from build123d import *

# Parameters (mm, degrees)
F1_DEPTH = 25.908
F2_W     = 84.75497365
F2_H     = 46.1407359689
F3_DEPTH = 35.306
F4_W     = 85.4094512761
F4_H     = 12.4350916594
F4_H_2   = 13.7440478429
F5_DEPTH = 44.45
F6_W     = 18.3254014701
F6_H     = 12.4350916594
F6_W_2   = 17.998162657
F6_H_2   = 12.1078519151
F6_W_3   = 19.3071179092
F6_H_3   = 13.7440478429
F7_DEPTH = 58.674
F8_R     = 6.9031193851
F9_DEPTH = 43.942


with BuildPart() as f1:
    # F0 (on Top) → F1 (new body)
    with BuildSketch(Plane.XY):
        Polygon((-13.4168099612, 56.1196766794), (-42.8683459759, 56.1196766794), (-42.8683459759, -55.7961538434), (-13.4168099612, -55.7961538434), (-13.4168099612, -41.0703867674), (12.7623323351, -41.0703867674), (12.7623323351, -55.7961538434), (42.2138683498, -55.7961538434), (42.2138683498, 56.1196766794), (12.7623323351, 56.1196766794), (12.7623323351, 41.0666689277), (-13.4168099612, 41.0666689277), align=None)
    extrude(amount=F1_DEPTH)

    # F2 (on Top) → F3 (join)
    with BuildSketch(Plane.XY):
        with Locations((-0.4908591509, 0.3253789619)):
            Rectangle(F2_W, F2_H)
    extrude(amount=F3_DEPTH)

    # F4 (on Top) → F5 (join)
    with BuildSketch(Plane.XY):
        with Locations((-0.4908572882, 17.1782011166)):
            Rectangle(F4_W, F4_H)
        with Locations((-0.4908572882, -15.5457244255)):
            Rectangle(F4_W, F4_H_2)
    extrude(amount=F5_DEPTH)

    # F6 (on Top) → F7 (join)
    with BuildSketch(Plane.XY):
        with Locations((-33.7056452408, 17.1782011166)):
            Rectangle(F6_W, F6_H)
        with Locations((33.2147870213, 17.3418209888)):
            Rectangle(F6_W_2, F6_H_2)
        with Locations((-33.8692646474, -15.5457244255)):
            Rectangle(F6_W_3, F6_H_3)
        with Locations((33.2147870213, -15.5457244255)):
            Rectangle(F6_W_2, F6_H_3)
    extrude(amount=F7_DEPTH)

    # F8 (on Top) → F9 (cut)
    with BuildSketch(Plane.XY):
        with Locations((6.05578674, 0)):
            Circle(F8_R)
    extrude(amount=F9_DEPTH, mode=Mode.SUBTRACT)


solid = f1.part
Check sheet for the modelled part. Datum: model origin and axes. Units: mm. A direction names the side the tool comes from. Round coordinates to 2 decimals unless told otherwise and drop trailing zeros. Order: outer loops, then holes, each group sorted by start corner. A loop starts at its lowest first (then second) coordinate and runs counter-clockwise, first axis right, second up.
(1) Go/stop test with flat-tipped pins: P1, Ø10, axis at x = 11, z = 14, coming from the +Y side; P2, Ø21.5, axis at x = 12.5, y = 2, coming from the +Z side; P3, Ø6, axis at y = 19.5, z = 33, coming from the -X side; P4, Ø16.5, axis at y = 48, z = 13.5, coming from the -X side. Record where each tip stops, or that it passes through.
(2) Cross-section at C-C, the plane x = 34. Enter the section's corners in (y, z), and give its area (3 significant figures).
(3) Cross-section at A-A, the plane y = 0. Enter the section's corners in (x, z), and give its area (3 significant figures).
(4) Cross-section at D-D, the plane z = 11.5. Enter the section's corners in (x, y), and give its area (3 significant figures).
(5) Scan lines: probe 1 along Y at (x, z) = (32, 38); probe 2 along X at (y, z) = (0, 17); probe 3 along Z at (x, y) = (21.5, 40.5). Record each from-to range of solid material in increasing order.
(6) Access from +Z, -Z, +X, -X, +Y, -Y to the whole of each face (thin tool, end or side, straight path). Record for faces 1 (the flat face through (-42.868, 1, 17)), 2 (the flat face through (12.762, -48, 13)), 3 (the flat face through (-42.868, 17, 51)), 4 (the flat face through (33, 11.288, 51)).
(7) Cross-section at B-B, the plane z = 47.5. Enter the section's corners in (x, y), and give its area (3 significant figures).
(8) Draft check along X on faces 5 (the flat face through (24.216, 17, 51)), 6 (the flat face through (-42.868, -39, 13)), 7 (the flat face through (-1, 1, 0)). Enter one of: pulls with the +X half, pulls with the -X half, needs draft (parallel to the pull), parting line crosses it, or undercut.
Check sheet entries:
1. P1: stops at y = 56.12
1. P2: stops at z = 44.45
1. P3: stops at x = -43.2
1. P4: stops at x = -42.87
2. outline: (-55.8, 0) - (56.12, 0) - (56.12, 25.91) - (23.4, 25.91) - (23.4, 58.67) - (11.29, 58.67) - (11.29, 44.45) - (10.96, 44.45) - (10.96, 35.31) - (-8.67, 35.31) - (-8.67, 58.67) - (-22.42, 58.67) - (-22.42, 35.31) - (-22.74, 35.31) - (-22.74, 25.91) - (-55.8, 25.91) - close
2. area: 3,940 mm2
3. outline: (-42.87, 0) - (-0.85, 0) - (-0.85, 35.31) - (-42.87, 35.31) - close; (12.96, 0) - (42.21, 0) - (42.21, 25.91) - (41.89, 25.91) - (41.89, 35.31) - (12.96, 35.31) - close
3. area: 2,510 mm2
4. outline: (-43.52, -22.42) - (-42.87, -22.42) - (-42.87, -55.8) - (-13.42, -55.8) - (-13.42, -41.07) - (12.76, -41.07) - (12.76, -55.8) - (42.21, -55.8) - (42.21, 56.12) - (12.76, 56.12) - (12.76, 41.07) - (-13.42, 41.07) - (-13.42, 56.12) - (-42.87, 56.12) - (-42.87, 23.4) - (-43.2, 23.4) - (-43.2, 10.96) - (-42.87, 10.96) - (-42.87, -8.67) - (-43.52, -8.67) - close; hole circle Ø13.81 at (6.06, 0)
4. area: 8,610 mm2
5. probe 1: y = -22.42 to -8.67, 10.96 to 23.4
5. probe 2: x = -42.87 to -0.85, 12.96 to 42.21
5. probe 3: z = 0 to 25.91
6. face 1: +Z, -Z, -X
6. face 2: +Z, -Z, -Y
6. face 3: +Z, -X, +Y
6. face 4: +Z, +X
7. outline: (-43.52, -22.42) - (-24.22, -22.42) - (-24.22, -8.67) - (-43.52, -8.67) - close; (-42.87, 10.96) - (-24.54, 10.96) - (-24.54, 23.4) - (-42.87, 23.4) - close; (24.22, -22.42) - (42.21, -22.42) - (42.21, -8.67) - (24.22, -8.67) - close; (24.22, 11.29) - (42.21, 11.29) - (42.21, 23.4) - (24.22, 23.4) - close
7. area: 959 mm2
8. face 5: undercut
8. face 6: pulls with the -X half
8. face 7: needs draft
